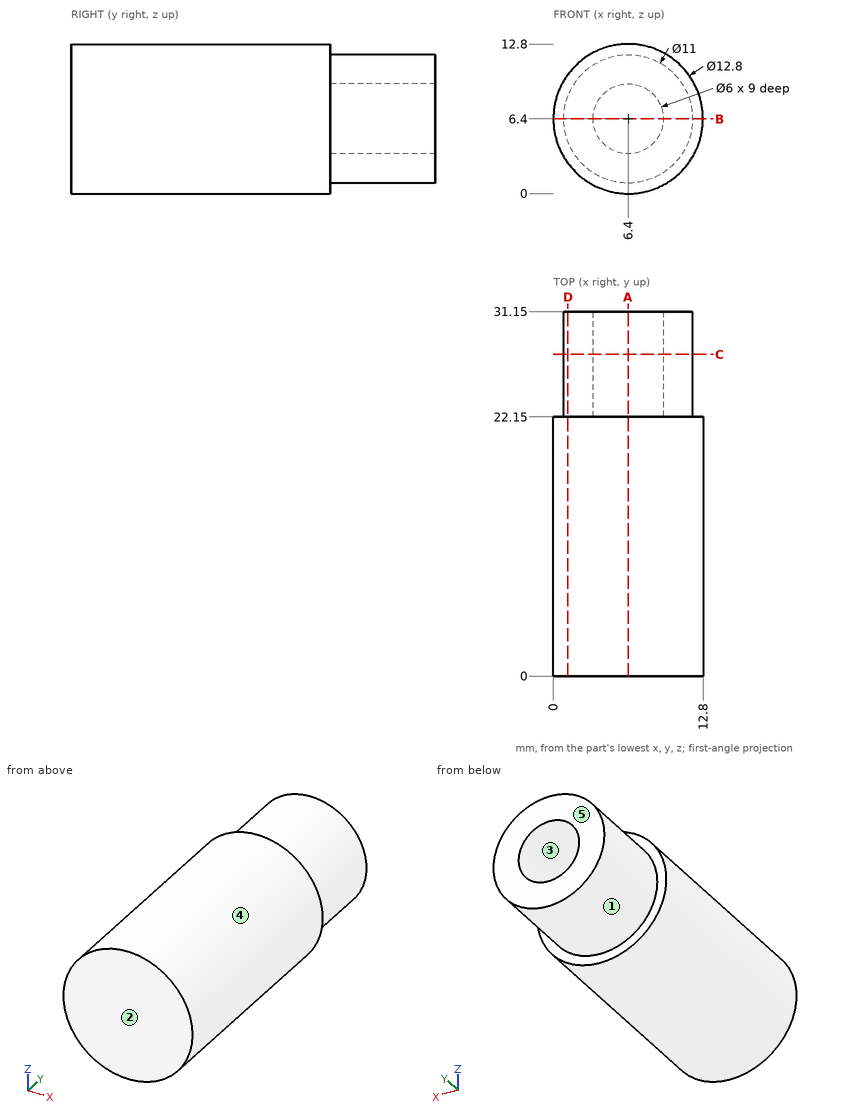
Geometry: see drawing. Coordinates: mm, zero at the bounding-box minimum. A direction names the side the tool comes from. Coordinates: 2 decimals unless noted, no trailing zeros. Order: outer loops, then holes, each group sorted by start corner. A loop starts at its lowest first (then second) coordinate and runs counter-clockwise, first axis right, second up. Notation, with made-up numbers: (41.25, 26) - (93.25, 26) arc R31 cw to (93.25, 59) - close; hole circle Ø10 at (4.5, 66). An arc over 180 degrees is marked (long way). Return JSON: item names as keys, results as strings.
Q1. Cut plane B-B (z = 6.4). Return loops of the section in (x, y), then the cut area to 3 significant figures.
The answers:
{"outline": "(0, 0) - (12.8, 0) - (12.8, 22.15) - (11.9, 22.15) - (11.9, 31.15) - (9.4, 31.15) - (9.4, 22.15) - (3.4, 22.15) - (3.4, 31.15) - (0.9, 31.15) - (0.9, 22.15) - (0, 22.15) - close", "area": "329 mm2"}
Q2. Cut plane C-C (y = 27.5). Return loops of the section in (x, z).
The answers:
{"outline": "circle Ø11 at (6.4, 6.4); hole circle Ø6 at (6.4, 6.4)"}
Q3. Ray query, probe 1 along Z at (x, y) = (6.4, 24.5); probe 2 along Y at (x, z) = (8.5, 12); probe 3 along Z at (x, y) = (4.5, 23). Return the intervals inside material, ascending.
The answers:
{"probe 1": "z = 0.9 to 3.4, 9.4 to 11.9", "probe 2": "y = 0 to 22.15", "probe 3": "z = 1.24 to 4.08, 8.72 to 11.56"}
Q4. Cut plane D-D (x = 1.25). Return loops of the section in (y, z).
The answers:
{"outline": "(0, 2.6) - (22.15, 2.6) - (22.15, 4.47) - (31.15, 4.47) - (31.15, 8.33) - (22.15, 8.33) - (22.15, 10.2) - (0, 10.2) - close"}
Q5. Draft query along Z for the marked faces 3, 4 and 5. Return one class per face: +Z half, -Z half, draft (parallel to the pull), parting line (faces both ways), or undercut.
The answers:
{"face 3": "undercut", "face 4": "parting line", "face 5": "draft"}
Q6. Cut plane A-A (x = 6.4). Return loops of the section in (y, z), then the cut area to 3 significant figures.
The answers:
{"outline": "(0, 0) - (22.15, 0) - (22.15, 0.9) - (31.15, 0.9) - (31.15, 3.4) - (22.15, 3.4) - (22.15, 9.4) - (31.15, 9.4) - (31.15, 11.9) - (22.15, 11.9) - (22.15, 12.8) - (0, 12.8) - close", "area": "329 mm2"}
Q7. Access query for the marked faces 1 and 2. Directions: +Z, -Z, +X, -X, +Y, -Y. A direction counts if a zero-diameter tool reaches every point of the face in a straight line with its end or side. Return the directions, or none.
The answers:
{"face 1": "+Y", "face 2": "+Z, -Z, +X, -X, -Y"}
Q8. First-contact query: pin 1 (5 mm diameter, centred on x = 7.5, z = 8, fed in from +Y); pin 2 (3 mm diameter, centred on x = 6.5, y = 25.5, fed in from +Z); pin 3 (4 mm diameter, centred on x = 2, y = 8.5, fed in from +Z); pin 4 (5.5 mm diameter, centred on x = 6.4, z = 6.4, fed in from +Y). Flat tips, straight axial feed; report the tip coordinate or a pass-through.
The answers:
{"pin 1": "stops at y = 31.15", "pin 2": "stops at z = 11.9", "pin 3": "stops at z = 12.33", "pin 4": "stops at y = 22.15"}
